Autodesk Inventor part; units mm, degrees
ref_plane "YZ Plane" through (0, 0, 0) normal (1, 0, 0) x (0, 1, 0)
ref_plane "XZ Plane" through (0, 0, 0) normal (0, 1, 0) x (-1, 0, 0)
ref_plane "XY Plane" through (0, 0, 0) normal (0, 0, 1) x (1, 0, 0)
sketch "Sketch1" plane through (0, 0, 0) normal (0, 1, 0) x (-1, 0, 0)
  line L0 (-7.5, -12.5) -> (7.5, -12.5)
  line L1 (7.5, -12.5) -> (7.5, 12.5)
  line L2 (7.5, 12.5) -> (-7.5, 12.5)
  line L3 (-7.5, 12.5) -> (-7.5, -12.5)
  line L4 (-7.5, -12.5) -> (7.5, 12.5) construction
  line L5 (7.5, -12.5) -> (-7.5, 12.5) construction
  point P0 (0, 0)
  dimension "d0" = 15
  dimension "d1" = 25
extrude "Extrusion1" add sketch "Sketch1" along normal blind 8
sketch "Sketch2" plane through (7.5, 0, -12.5) normal (1, 0, 0) x (0, 0, -1)
  line L0 (-25, 0) -> (-25, 8)
  line L1 (-25, 8) -> (0, 8)
  point P0 (-12.5, 0)
  point P1 (-21, 4)
  point P2 (-25, 2)
  point P3 (-25, 6)
  point P4 (-23, 8)
  dimension "d5" = 4
  dimension "d6" = 4
hole "Hole1" at (7.5, 4, 8.5) direction (-1, 0, 0) diameter 4 end through all
sketch "Sketch4" plane through (7.5, 0, -12.5) normal (1, 0, 0) x (0, 0, -1)
  point P0 (-12.5, 0)
sketch "Sketch5" plane through (7.5, 0, 12.5) normal (1, 0, 0) x (0, 0, -1)
  line L0 (25, 0) -> (0, 0)
  line L1 (0, 0) -> (8, 0)
  line L2 (8, 0) -> (8, -17)
  line L3 (8, -17) -> (0, -17)
  line L4 (0, -17) -> (0, 0)
  point P0 (12.5, 0)
  dimension "d20" = 8
  dimension "d21" = 17
extrude "Extrusion3" add sketch "Sketch5" against normal blind 15
fillet "Fillet3" radius 2 3 edges at (0, -17, 12.5) (0, -17, 4.5) (0, 8, 12.5)
sketch "Sketch6" plane through (7.5, 0, -12.5) normal (1, 0, 0) x (0, 0, -1)
  line L0 (0, 8) -> (-23, 8)
  line L1 (0, 8) -> (-8, 8)
  line L2 (-8, 8) -> (-8, 61.5)
  line L3 (-8, 61.5) -> (0, 61.5)
  line L4 (0, 61.5) -> (0, 8)
  point P0 (-12.5, 0)
  dimension "d25" = 8
  dimension "d26" = 53.5
extrude "Extrusion4" add sketch "Sketch6" against normal blind 15
fillet "Fillet4" radius 2 3 edges at (0, 0, -12.5) (0, 61.5, -4.5) (0, 61.5, -12.5)
sketch "Sketch7" plane through (7.5, -15, 4.5) normal (1, 0, 0) x (0, 0, -1)
  line L0 (9, 23) -> (9, 74.5)
  line L1 (17, 76.5) -> (9, 76.5)
  line L2 (9, 76.5) -> (9, 66.5)
  line L3 (9, 66.5) -> (17, 66.5)
  line L4 (17, 66.5) -> (17, 76.5)
  line L5 (11, 76.5) -> (15, 76.5)
  point P0 (4.5, 15)
  dimension "d30" = 10
  dimension "d43" = 0
extrude "Extrusion5" cut sketch "Sketch7" against normal blind 7.5
sketch "Sketch8" plane through (0, -15, 4.5) normal (1, 0, 0) x (0, 0, -1)
  line L0 (17, 74.5) -> (17, 66.5)
  line L1 (11, 76.5) -> (15, 76.5)
  point P0 (4.5, 15)
  point P1 (13, 71.5)
  dimension "d33" = 4
  dimension "d34" = 5
hole "Hole2" at (0, 56.5, -8.5) direction (-1, 0, 0) diameter 3 end through all
fillet "Fillet5" radius 2 1 edges at (3.75, 51.5, -4.5)
properties part number "Lever"
CAD build for the part. Positions are in the model's coordinates, mm. A direction names the side the tool comes from. Coordinates: 2 decimals unless noted, no trailing zeros. Loops run counter-clockwise (first coordinate to the right, second up) from the corner with the lowest first, then second, coordinate; pieces in that order, holes last. Notation, with made-up numbers: (25.5, 44.25) - (68.5, 44.25) arc R23 ccw to (68.5, 66.25) - close; hole circle Ø9 at (-39.75, 54.5). An arc over 180 degrees is marked (long way). Write item = value, one per line. Start each with the question number.
Q1. Cut at B-B, the plane y = 4. List the corners of the cut face in (x, z), then the cut area to 3 significant figures.
Q2. Drill centre lines: L1, parallel to Z at x = -4.25, y = 56.5; L2, parallel to Y at x = -4, z = -8.5; L3, parallel to Z at x = -3.75, y = 4. Where is each one in solid material? Low to high.
Q3. Cut at D-D, the plane x = 4.25. List the corners of the cut face in (y, z), then the cut area to 3 significant figures.
Q4. Cut at A-A, the plane z = -8.5. List the corners of the cut face in (x, y).
Q5. Cut at C-C, the plane x = -2.75. List the corners of the cut face in (y, z).
Q6. Flat gauge pins, fed straight in: pin 1 Ø6 at (x, y) = (3.5, -5) entering from -Z; pin 2 Ø3 at (x, z) = (-0.5, 0.5) entering from -Y; pin 3 Ø1.5 at (x, y) = (-3, 36.5) entering from +Z. Where does each tip first touch, or does it go through?
Q7. Which spindle directions (+Z, -Z, +X, -X, +Y, -Y) get a long thin tool onto all of the face, cutting with end or side? Do faces 1 (the flat face through (0, 33, -4.5)), 2 (the flat face through (0, -7, 4.5)), 3 (the cylindrical face through (3.7, 50.9, -5.07)). Say none if no direction does.
Q8. Pull direction Y, two halves, no side cores. Call faces 4 (the flat face through (-4, 61.5, -8)), 5 (the flat face through (0, 55.6, -6.7)), 6 (the cylindrical face through (-0.11, -16.4, 5.07)), 7 (the cylindrical face through (-3.802, 55.013, -8.305)): pulls with the +Y half, pulls with the -Y half, needs draft (parallel to the pull), parting line crosses it, or undercut.
Computed:
q1.outline = (-7.5, -12.5) - (7.5, -12.5) - (7.5, 6.5) - (-7.5, 6.5) - close; (-7.5, 10.5) - (7.5, 10.5) - (7.5, 12.5) - (-7.5, 12.5) - close
q1.area = 315 mm²
q2.L1 = -12.5 to -10, -7 to -4.5
q2.L2 = 0 to 55, 58 to 61.5
q2.L3 = -12.5 to 6.5, 10.5 to 12.5
q3.outline = (-17, 6.5) arc R2 ccw to (-15, 4.5) - (0, 4.5) - (0, -10.5) arc R2 ccw to (2, -12.5) - (51.5, -12.5) - (51.5, -6.5) arc R2 ccw to (49.5, -4.5) - (8, -4.5) - (8, 10.5) arc R2 ccw to (6, 12.5) - (-15, 12.5) arc R2 ccw to (-17, 10.5) - close; hole circle Ø4 at (4, 8.5)
q3.area = 667 mm²
q4.outline = (-7.5, 0) - (7.5, 0) - (7.5, 51.5) - (0, 51.5) - (0, 55) - (-7.5, 55) - close; (-7.5, 58) - (0, 58) - (0, 61.5) - (-7.5, 61.5) - close
q5.outline = (-17, 6.5) arc R2 ccw to (-15, 4.5) - (0, 4.5) - (0, -10.5) arc R2 ccw to (2, -12.5) - (59.5, -12.5) arc R2 ccw to (61.5, -10.5) - (61.5, -6.5) arc R2 ccw to (59.5, -4.5) - (8, -4.5) - (8, 10.5) arc R2 ccw to (6, 12.5) - (-15, 12.5) arc R2 ccw to (-17, 10.5) - close; hole circle Ø4 at (4, 8.5); hole circle Ø3 at (56.5, -8.5)
q6.pin_1 = 4.5
q6.pin_2 = 0
q6.pin_3 = -4.5
q7.face_1 = +Z, +X, -X, +Y
q7.face_2 = -Z, +X, -X, -Y
q7.face_3 = +Z, +X, +Y
q8.face_4 = pulls with the +Y half
q8.face_5 = needs draft
q8.face_6 = pulls with the -Y half
q8.face_7 = undercut
